Build history of the part. All positions in model axes, mm. A direction names the side the tool comes from. Give positions to 0.01 mm unless a question says otherwise; leave off trailing zeros. Loops run counter-clockwise (first coordinate to the right, second up) from the corner with the lowest first, then second, coordinate; pieces in that order, holes last. Notation, with made-up numbers: (-6.75, 8) -> (39.25, 8) arc R20 cw to (39.25, 37) -> close; hole circle Ø9 at (-4.75, 6.25). An arc over 180 degrees is marked (long way). Answer as a JSON object with one key per item and string values. Group by question number.
Q1. Two-plate mould, pull along X, no slides. Class faces 3 (the flat face through (50.5, 25, 44)), 4 (the cylindrical face through (1.804, 48.789, 45.63)), 5 (the conical face through (9.64, 8.95, 84.06)): pulls with the +X half, pulls with the -X half, needs draft (parallel to the pull), parting line crosses it, or undercut.
Q2. Tool access for faces 1 (the cylindrical face through (44.3, 41.8, 87.1)), 2 (the cylindrical face through (6.428, 46.447, 41.574)): list every direction of +Z, -Z, +X, -X, +Y, -Y with a clear straight run to the whole face (end or side of a thin tool).
Q3. Wall check: probe 1 along X at (y, z) = (7.75, 44.5); probe 2 along X at (y, z) = (7.75, 86.2). Give the ranges that are in metal, low to high. Write a range as from..to.
Q4. Drop flat-ended pins along their axis: pin 1 (4 mm diameter, centred on x = 7.75, y = 7.75, fed in from +Z); pin 2 (5.5 mm diameter, centred on x = 42.25, y = 42.25, fed in from -Z); pin 3 (7 mm diameter, centred on x = 7.75, y = 42.25, fed in from -Z); pin 4 (5 mm diameter, centred on x = 42.25, y = 7.75, fed in from -Z). Give the stop position or say it passes through.
Q5. Band-saw the part on A-A, the plane y = 42.25. Write the cut outline in (x, z).
Q6. Band-saw the part on C-C, the plane z = 28. Write the cut outline in (x, y).
Q7. Band-saw the part on D-D, the plane z = 9. Write the cut outline in (x, y), plus the area to 3 significant figures.
Autodesk Fusion 360 part; units mm, degrees
sketch "Skizze1" plane through (0, 0, 0) normal (0, 0, 1) x (1, 0, 0)
  line L0 (0, 0) -> (50.5, 0)
  line L1 (50.5, 0) -> (50.5, 50.5)
  line L2 (50.5, 50.5) -> (0, 50.5)
  line L3 (0, 50.5) -> (0, 0)
  line L4 (50.5, 0) -> (50.5, 5)
  line L5 (50.5, 5) -> (50.5, 8.5)
  line L6 (50.5, 8.5) -> (50.5, 13.5)
  circle A0 centre (25, 25) radius 12.7
  line L7 (42.25, 42.25) -> (7.75, 42.25)
  line L8 (7.75, 42.25) -> (7.75, 7.75)
  line L9 (7.75, 7.75) -> (42.25, 7.75)
  line L10 (42.25, 7.75) -> (42.25, 42.25)
  line L11 (42.25, 42.25) -> (7.75, 7.75) construction
  line L12 (7.75, 42.25) -> (42.25, 7.75) construction
  point P0 (25, 25)
  dimension "d1" = 50.5
  dimension "d2" = 50.5
  dimension "d17" = 25.4
  dimension "d18" = 34.5
  dimension "d19" = 34.5
extrude "Extrusion1" add sketch "Skizze1" along normal blind 90 contours L0 L1 L2 L3 L4 L5 L6 | A0 | L7 L8 L9 L10
extrude "Extrusion2" cut sketch "Skizze1" along normal blind 15 contours A0
chamfer "Fase1" distance 2.5 distance2 15 1 edges at (13.1594, 20.4075, 0) measured on face at (25.483, 46.2215, 0)
sketch "Skizze2" plane through (0, 0, 0) normal (0, 0, -1) x (1, 0, 0)
  line L0 (0, 0) -> (0, -50.5)
  line L1 (0, -50.5) -> (50.5, -50.5)
  line L2 (50.5, -50.5) -> (50.5, 0)
  line L3 (50.5, 0) -> (0, 0)
  circle A0 centre (25, -25) radius 15.2
  line L4 (42.25, -7.75) -> (7.75, -7.75)
  line L5 (7.75, -7.75) -> (7.75, -42.25)
  line L6 (7.75, -42.25) -> (42.25, -42.25)
  line L7 (42.25, -42.25) -> (42.25, -7.75)
  line L8 (42.25, -7.75) -> (7.75, -42.25) construction
  line L9 (7.75, -7.75) -> (42.25, -42.25) construction
  point P0 (25, -25)
  dimension "d26" = 34.5
  dimension "d27" = 34.5
hole "Bohrung1" at (7.75, 7.75, 0) at (7.75, 42.25, 0) at (42.25, 42.25, 0) at (42.25, 7.75, 0) direction (0, 0, 1) diameter 8.8 depth 82 tip angle 180
hole "Bohrung2" at (7.75, 42.25, 82) direction (0, 0, 1) diameter 4.2 depth 82 tip angle 180 countersink diameter 8.6 countersink angle 90
hole "Bohrung3" at (7.75, 7.75, 82) direction (0, 0, 1) diameter 4.2 depth 82 tip angle 180 countersink diameter 8.6 countersink angle 90
hole "Bohrung4" at (42.25, 7.75, 82) direction (0, 0, 1) diameter 4.2 depth 82 tip angle 180 countersink diameter 8.6 countersink angle 90
hole "Bohrung5" at (42.25, 42.25, 82) direction (0, 0, 1) diameter 4.2 depth 82 tip angle 180 countersink diameter 8.6 countersink angle 90
fillet "Fillet3" radius 6 1 edges at (0, 50.5, 45)
fillet "Fillet4" radius 1 3 edges at (0, 0, 45) (50.5, 0, 45) (50.5, 50.5, 45)
Worked answers:
{
 "1": {"face 3": "pulls with the +X half", "face 4": "pulls with the -X half", "face 5": "undercut"},
 "2": {"face 1": "+Z, -Z", "face 2": "-Z"},
 "3": {"probe 1": "0..3.35, 12.15..37.85, 46.65..50.5", "probe 2": "0..5.65, 9.85..40.15, 44.35..50.5"},
 "4": {"pin 1": "through", "pin 2": "z = 83.55", "pin 3": "z = 82.8", "pin 4": "z = 83.8"},
 "5": {"outline": "(0, 0) -> (3.35, 0) -> (3.35, 82) -> (3.45, 82) -> (5.65, 84.2) -> (5.65, 90) -> (0, 90) -> close; (9.85, 84.2) -> (12.05, 82) -> (12.15, 82) -> (12.15, 0) -> (37.85, 0) -> (37.85, 82) -> (37.95, 82) -> (40.15, 84.2) -> (40.15, 90) -> (9.85, 90) -> close; (44.35, 84.2) -> (46.55, 82) -> (46.65, 82) -> (46.65, 0) -> (50.5, 0) -> (50.5, 90) -> (44.35, 90) -> close"},
 "6": {"outline": "(0, 1) arc R1 ccw to (1, 0) -> (49.5, 0) arc R1 ccw to (50.5, 1) -> (50.5, 49.5) arc R1 ccw to (49.5, 50.5) -> (6, 50.5) arc R6 ccw to (0, 44.5) -> close; hole circle Ø8.8 at (7.75, 7.75); hole circle Ø8.8 at (7.75, 42.25); hole circle Ø8.8 at (42.25, 7.75); hole circle Ø8.8 at (42.25, 42.25)"},
 "7": {"outline": "(0, 1) arc R1 ccw to (1, 0) -> (49.5, 0) arc R1 ccw to (50.5, 1) -> (50.5, 49.5) arc R1 ccw to (49.5, 50.5) -> (6, 50.5) arc R6 ccw to (0, 44.5) -> close; hole circle Ø8.8 at (7.75, 7.75); hole circle Ø8.8 at (7.75, 42.25); hole circle Ø27.4 at (25, 25); hole circle Ø8.8 at (42.25, 7.75); hole circle Ø8.8 at (42.25, 42.25)", "area": "1,710 mm2"}
}
